Part model, mm, in its own coordinate system. A direction names the side the tool comes from. Coordinates: 2 decimals unless noted, no trailing zeros. Write each loop counter-clockwise with the first axis right and the second up, starting at its lowest first coordinate (ties: lowest second). Pieces come first, ordered by that corner, then holes. Notation, with made-up numbers: (-3.75, -35) -> (38.25, -35) arc R9 ccw to (38.25, -30) -> close; hole circle Ø10 at (66.5, 39). An arc over 180 degrees is marked (long way). Write item = value, one per line. Start each with the question number.
Q1. Pull direction X, two halves, no side cores. Call faces 4 (the flat face through (-2, -13.5, 2)), 5 (the flat face through (0.2, -10, 3)), 6 (the cylindrical face through (-2.15, -0.09, 1.97)), 7 (the flat face through (5, -4, 2)): released by +X, released by -X, zero draft, split by the parting line, or undercut.
Q2. Tool access for faces 1 (the cylindrical face through (-1.236, -4.337, 0.592)), 2 (the flat face through (1, -4, 4)), 3 (the flat face through (-3, -7, 2.8)): list every direction of +Z, -Z, +X, -X, +Y, -Y with a clear straight run to the whole face (end or side of a thin tool).
Q3. Band-saw the part on C-C, the plane x = -3. List the corners of the cut face in (y, z).
Q4. Pin check, flat tips, straight feed: P1, Ø2.5, axis at x = 0, y = 0, coming from the -Z side; P2, Ø1, axis at x = 4, z = 2, coming from the +Y side; P3, Ø2, axis at y = 2, z = 2.5, coming from the +X side; P4, Ø4, axis at x = -2, y = -9, coming from the -Z side. Stop position of each tip, or through.
Q5. Band-saw the part on D-D, the plane y = -5.25. List the corners of the cut face in (x, z).
Q6. Probe line 1 (Y direction, x = 0, z = 1.25); line 2 (Z direction, x = -2.5, y = -5.25); line 3 (Y direction, x = -3, z = 2.2). List the from-to ranges inside material, lowest first.
Q7. Band-saw the part on B-B, the plane y = -9. List the corners of the cut face in (x, z), plus the area to 3 significant figures.
Autodesk Inventor part; units mm, degrees
ref_plane "YZ Plane" through (0, 0, 0) normal (1, 0, 0) x (0, 1, 0)
ref_plane "XZ Plane" through (0, 0, 0) normal (0, 1, 0) x (-1, 0, 0)
ref_plane "XY Plane" through (0, 0, 0) normal (0, 0, 1) x (1, 0, 0)
sketch "Boceto39" plane through (0, 0, 0) normal (0, 0, 1) x (1, 0, 0)
  circle A0 centre (0, 0) radius 2.15
  line L0 (-5, 5) -> (0, 5)
  line L1 (5, 0) -> (5, -13.5)
  line L2 (5, -13.5) -> (-5, -13.5)
  line L3 (-5, -13.5) -> (-5, 5)
  arc A1 (5, 0) -> (0, 5) centre (0, 0) ccw
  dimension "d373" = 4.3
  dimension "d374" = 5
  dimension "d375" = 10
  dimension "d376" = 18.5
extrude "Extrusión13" add sketch "Boceto39" along normal blind 4
sketch "Boceto40" plane through (-5, -13.5, 0) normal (-1, 0, 0) x (0, 0, 1)
  line L0 (0, 0) -> (0, 18.5) construction
  line L1 (0, 0) -> (4, 0) construction
  line L2 (4, 18.5) -> (4, 0) construction
  line L3 (0, 18.5) -> (4, 18.5) construction
  line L4 (0, 4) -> (1.2, 4)
  line L5 (1.2, 4) -> (1.2, 1.7)
  line L6 (1.2, 1.7) -> (0, 1.7)
  line L7 (0, 1.7) -> (0, 4)
  line L8 (4, 18.5) -> (4, 0)
  line L9 (4, 4) -> (2.8, 4)
  line L10 (2.8, 4) -> (2.8, 1.7)
  line L11 (2.8, 1.7) -> (4, 1.7)
  line L12 (4, 1.7) -> (4, 4)
  point P0 (0, 13.5)
  dimension "d379" = 1.7
  dimension "d380" = 2.3
  dimension "d381" = 1.2
extrude "Extrusión14" cut sketch "Boceto40" against normal blind 5.2
sketch "Boceto41" plane through (0, 0, 0) normal (0, 0, -1) x (-1, 0, 0)
  line L0 (-0.2, -11.8) -> (-0.2, -9.5) construction
  line L1 (5, -9.5) -> (5, 5) construction
  arc A0 (5, -0.7273) -> (-0.2, -9.5) centre (9.8, -9.5) ccw
  line L2 (5, 5) -> (5, -9.5) construction
  line L3 (-0.2, -9.5) -> (5, -9.5)
  line L4 (5, -9.5) -> (5, -0.7273)
  point P0 (0, 0)
  dimension "d384" = 10
extrude "Extrusión15" cut sketch "Boceto41" against normal up to surface (1.2 mm away)
sketch "Boceto42" plane through (0, 0, 4) normal (0, 0, 1) x (1, 0, 0)
  line L0 (-5, -9.5) -> (0.2, -9.5)
  line L1 (0.2, -9.5) -> (0.2, -11.8) construction
  line L2 (0.2, -11.8) -> (-5, -11.8) construction
  line L3 (-5, -11.8) -> (-5, -13.5) construction
  line L4 (-5, -13.5) -> (5, -13.5) construction
  line L5 (5, -13.5) -> (5, 0) construction
  arc A0 (5, 0) -> (0, 5) centre (0, 0) ccw construction
  line L6 (0, 5) -> (-5, 5) construction
  line L7 (-5, 5) -> (-5, -9.5) construction
  circle A1 centre (0, 0) radius 2.15 construction
  line L8 (-5, -0.7273) -> (-5, -11.8) construction
  arc A2 (0.2, -9.5) -> (-5, -0.7273) centre (-9.8, -9.5) ccw
  line L9 (0.2, -9.5) -> (0.2, -11.8) construction
  line L10 (-5, -11.8) -> (0.2, -11.8) construction
  line L11 (-5, -11.8) -> (-5, -9.5)
  line L12 (-5, -9.5) -> (-5, -0.7273)
  line L13 (-5, -9.5) -> (0.2, -9.5)
  line L14 (-5, -9.5) -> (0.2, -9.5)
  line L15 (0.2, -9.5) -> (0.2, -11.8)
  line L16 (-5, -0.7273) -> (-5, -11.8)
  arc A3 (0.2, -9.5) -> (-5, -0.7273) centre (-9.8, -9.5) ccw
extrude "Extrusión16" cut sketch "Boceto42" against normal up to surface (1.2 mm away)
fillet "Empalme44" radius 5 1 edges at (-5, 5, 2)
fillet "Empalme45" radius 5 1 edges at (5, -13.5, 2)
fillet "Empalme46" radius 1.5 1 edges at (-5, -13.5, 2)
fillet "Empalme46" radius 0.5 2 edges at (0.2, -11.8, 0.6) (0.2, -11.8, 3.4)
properties part number "PP-I3D-0001"
Ans:
q1.face_4 = zero draft
q1.face_5 = released by -X
q1.face_6 = undercut
q1.face_7 = released by +X
q2.face_1 = -Z, -X
q2.face_2 = +Z, +X, -X, +Y, -Y
q2.face_3 = +Z, -X
q3.outline = (-13.5, 0) -> (-11.8, 0) -> (-11.8, 1.2) -> (-2.17, 1.2) -> (-2.17, 0) -> (4, 0) -> (4, 4) -> (-2.17, 4) -> (-2.17, 2.8) -> (-11.8, 2.8) -> (-11.8, 4) -> (-13.5, 4) -> close
q4.P1 = through
q4.P2 = 3.57
q4.P3 = 4.9
q4.P4 = 1.2
q5.outline = (-5, 1.2) -> (-0.75, 1.2) -> (-0.75, 0) -> (5, 0) -> (5, 4) -> (-0.75, 4) -> (-0.75, 2.8) -> (-5, 2.8) -> close
q6.line_1 = -13.5 to -2.15, 2.15 to 5
q6.line_2 = 1.2 to 2.8
q6.line_3 = -13.5 to 4
q7.outline = (-5, 1.2) -> (0.19, 1.2) -> (0.19, 0) -> (4.97, 0) -> (4.97, 4) -> (0.19, 4) -> (0.19, 2.8) -> (-5, 2.8) -> close
q7.area = 27.4 mm2
